```python
from build123d import *

# Parameters (mm, degrees)
BASE_SKETCH_W         = 125
BASE_SKETCH_H         = 80
BASE_EXTRUDE_DEPTH    = 4
INSET_SKETCH_W        = 116.5
INSET_SKETCH_H        = 71.5
INSET_EXTRUDE_DEPTH   = 2
INNER_HOLE_SKETCH_W   = 28
INNER_HOLE_SKETCH_H   = 27
INNER_HOLE_CUT_DEPTH  = 12
OUTER_HOLE_SKETCH_W   = 44
OUTER_HOLE_SKETCH_H   = 31
OUTTER_HOLE_CUT_DEPTH = 2.5
MIDDLE_HOLE_SKETCH_W  = 38
MIDDLE_HOLE_SKETCH_H  = 31
MIDDLE_HOLE_CUT_DEPTH = 5
F_1_0MM_DOWEL_HOLE1_D = 1


with BuildPart() as part:
    # base sketch → base extrude (new body)
    with BuildSketch(Plane(origin=(0, 0, 0), x_dir=(1, 0, 0), z_dir=(0, 1, 0))):
        with Locations((62.5, 40)):
            Rectangle(BASE_SKETCH_W, BASE_SKETCH_H)
    extrude(amount=BASE_EXTRUDE_DEPTH)

    # inset sketch → inset extrude (add)
    with BuildSketch(Plane(origin=(0, 4, 0), x_dir=(1, 0, 0), z_dir=(0, 1, 0))):
        with Locations((62.5, 40)):
            Rectangle(INSET_SKETCH_W, INSET_SKETCH_H)
    extrude(amount=INSET_EXTRUDE_DEPTH)

    # inner hole sketch → inner hole cut (cut)
    with BuildSketch(Plane(origin=(0, 6, 0), x_dir=(1, 0, 0), z_dir=(0, 1, 0))):
        with Locations((96, 51.5)):
            Rectangle(INNER_HOLE_SKETCH_W, INNER_HOLE_SKETCH_H)
    extrude(amount=-INNER_HOLE_CUT_DEPTH, mode=Mode.SUBTRACT)

    # outer hole sketch → outter hole cut (cut)
    with BuildSketch(Plane(origin=(0, 6, 0), x_dir=(1, 0, 0), z_dir=(0, 1, 0))):
        with Locations((91, 51.5)):
            Rectangle(OUTER_HOLE_SKETCH_W, OUTER_HOLE_SKETCH_H)
    extrude(amount=-OUTTER_HOLE_CUT_DEPTH, mode=Mode.SUBTRACT)

    # middle hole sketch → middle hole cut (cut)
    with BuildSketch(Plane(origin=(0, 6, 0), x_dir=(1, 0, 0), z_dir=(0, 1, 0))):
        with Locations((94, 51.5)):
            Rectangle(MIDDLE_HOLE_SKETCH_W, MIDDLE_HOLE_SKETCH_H)
    extrude(amount=-MIDDLE_HOLE_CUT_DEPTH, mode=Mode.SUBTRACT)

    # Ø1.0mm Dowel Hole1 (through all)
    with Locations(Plane(origin=(123, 0, -78), x_dir=(0, 0, -1), z_dir=(0, -1, 0))):
        with Locations((0, 0), (-76, 0), (-76, -121), (0, -121)):
            Hole(F_1_0MM_DOWEL_HOLE1_D / 2)


solid = part.part
```
The listing builds one solid part. Answer for the finished solid, in the listing's coordinates (mm). A direction names the side the tool comes from. Coordinates: 2 decimals unless noted, no trailing zeros. Write each loop counter-clockwise with the first axis right and the second up, starting at its lowest first coordinate (ties: lowest second). Pieces come first, ordered by that corner, then holes. Notation, with made-up numbers: (21, -6.75) - (49, -6.75) arc R21 cw to (49, 3.25) - close; hole circle Ø4 at (-16, 19). An arc over 180 degrees is marked (long way). One line per item, written item: value.
1) Find section A-A (z = -63). Give the vertices of the cut face in (x, y), and give its area (3 significant figures).
Geometry check:
outline: (0, 0) - (82, 0) - (82, 1) - (75, 1) - (75, 3.5) - (69, 3.5) - (69, 6) - (4.25, 6) - (4.25, 4) - (0, 4) - close; (110, 0) - (125, 0) - (125, 4) - (120.75, 4) - (120.75, 6) - (113, 6) - (113, 1) - (110, 1) - close
area: 500 mm2
2) For a pull along X with two mould halves and no side action, classify faces 1 (the flat face through (62, 2, -80)), 2 (the flat face through (113, 4, -51)), 3 (the flat face through (0, 2, -39)) as pulls with the +X half, pulls with the -X half, needs draft (parallel to the pull), parting line crosses it, or undercut.
Geometry check:
face 1: needs draft
face 2: undercut
face 3: pulls with the -X half
3) A tool of negligible diameter and unlimited length cuts with its end or side. For faces 4 (the flat face through (91, 4, -67)), 5 (the flat face through (62, 2, 0)), from which of +Z, -Z, +X, -X, +Y, -Y can it reach the whole face along a straight path? Write none if from no direction.
Geometry check:
face 4: +Y
face 5: +Z, +X, -X, +Y, -Y
4) Find section C-C (z = -15). Give the vertices of the cut face in (x, y), and give its area (3 significant figures).
Geometry check:
outline: (0, 0) - (125, 0) - (125, 4) - (120.75, 4) - (120.75, 6) - (4.25, 6) - (4.25, 4) - (0, 4) - close
area: 733 mm2
5) Consider line 1 along Z through (x, y) = (123, 1.5); line 2 along X through (y, z) = (3, -78); line 3 along Z through (x, y) = (95, 3.6). Determine where each line is inside the solid, lowest interval first. Write a range as from..to.
Geometry check:
line 1: z = -80..-78.5, -77.5..-2.5, -1.5..0
line 2: x = 0..1.5, 2.5..122.5, 123.5..125
line 3: z = -80..-67, -36..0
6) Find section D-D (x = 56). Give the vertices of the cut face in (y, z).
Geometry check:
outline: (0, -80) - (4, -80) - (4, -75.75) - (6, -75.75) - (6, -4.25) - (4, -4.25) - (4, 0) - (0, 0) - close
7) Find section B-B (x = 91). Give the vertices of the cut face in (y, z).
Geometry check:
outline: (0, -80) - (4, -80) - (4, -75.75) - (6, -75.75) - (6, -67) - (1, -67) - (1, -65) - (0, -65) - close; (0, -38) - (1, -38) - (1, -36) - (6, -36) - (6, -4.25) - (4, -4.25) - (4, 0) - (0, 0) - close
8) Each of these flat-tipped pins is pushed along its axis until it touches: pin 1 Ø0.5 at (y, z) = (0.5, -46.5) entering from -X; pin 2 Ø3 at (x, z) = (72.5, -54) entering from +Y; pin 3 Ø1 at (x, y) = (67, 5) entering from +Z; pin 4 Ø0.6 at (y, z) = (5, -40.5) entering from +X. Where does it stop, or does it pass through?
Geometry check:
pin 1: stops at x = 0
pin 2: stops at y = 3.5
pin 3: stops at z = -4.25
pin 4: stops at x = 120.75
